from build123d import *

# Parameters (mm, degrees)
F0_W    = 7.5
F0_H    = 120
F4_SIZE = 4.99999


# Not quite as in the source:
# - a fillet or chamfer is up to 0.001 mm smaller than in the source, because OpenCascade refuses the exact size


with BuildPart() as f1:
    # F0 (on Front) → F1 (revolve)
    with BuildSketch(Plane.XZ):
        Polygon((0, 65), (0, 60), (7.5, 60), (17.5, 60), (17.5, 65), align=None)
    revolve(axis=Axis((0, 0, 0), (0, 0, -1)))

    # F0 (on Front) → F2 (revolve)
    with BuildSketch(Plane.XZ):
        with Locations((3.75, 0)):
            Rectangle(F0_W, F0_H)
    revolve(axis=Axis((0, 0, 0), (0, 0, -1)))

    # F0 (on Front) → F3 (revolve)
    with BuildSketch(Plane.XZ):
        Polygon((7.5, -60), (0, -60), (0, -65), (17.5, -65), (17.5, -60), align=None)
    revolve(axis=Axis((0, 0, 0), (0, 0, -1)))

    # F4 (size 5 in the source; OpenCascade refuses exactly that, so slightly less here)
    f4_edges = [f1.edges().sort_by_distance(p)[0] for p in [
        (-17.5, 0, 60),
        (-7.5, 0, 60),
    ]]
    chamfer(f4_edges, length=F4_SIZE)


solid = f1.part
Design review of the part built by this model. Coordinates are the model's own, in mm. A direction names the side the tool comes from. Give positions to 0.01 mm unless a question says otherwise; leave off trailing zeros. Write each loop counter-clockwise with the first axis right and the second up, starting at its lowest first coordinate (ties: lowest second). Pieces come first, ordered by that corner, then holes. Notation, with made-up numbers: M 62,42.5 L 121,42.5 A15 ccw 121,65.5 Z; hole C 50.25,33 d9. An arc over 180 degrees is marked long. Answer as a JSON object with one key per item and string values. Group by question number.
1) We need section C-C (z = 27). Give the boundary of the cut face in (x, y).
2) Clearance check with flat-ended pins moving along their axes: pin 1 Ø8 at (x, z) = (-5, 40) entering from +Y; pin 2 Ø1 at (y, z) = (0.5, 4.5) entering from -X; pin 3 Ø8 at (x, z) = (-3.5, 34.5) entering from -Y. State where each tip first meets the part, or that it passes through.
3) For line 1 along Z through (x, y) = (14.5, 9); line 2 along Z through (x, y) = (1, 12); line 3 along X through (y, z) = (-3, 17), list the stretches that pass through material, from the lowest coordinate up.
4) Tool access review of faces 1 (the face through (0, 8, -60)), 2 (the face through (0, 0, -65)): name each direction out of +Z, -Z, +X, -X, +Y, -Y from which nothing blocks a thin tool from reaching the whole face with its end or side.
5) Mouldability with a two-part tool opening along Z and no side actions: class faces 3 (the face through (-13.887, 10.648, -62.465)), 4 (the face through (-7.493, -0.33, -1.695)), 5 (the face through (0, 0, 65)) as released by +Z, released by -Z, zero draft, split by the parting line, or undercut.
Answer key:
{
 "1": {"outline": "C 0,0 d15"},
 "2": {"pin 1": "stops at y = 7.43", "pin 2": "stops at x = -7.5", "pin 3": "stops at y = -7.5"},
 "3": {"line 1": "z = -65 to -60, 64.57 to 65", "line 2": "z = -65 to -60, 59.54 to 65", "line 3": "x = -6.87 to 6.87"},
 "4": {"face 1": "none", "face 2": "-Z, +X, -X, +Y, -Y"},
 "5": {"face 3": "zero draft", "face 4": "undercut", "face 5": "released by +Z"}
}
